from build123d import *

# Parameters (mm, degrees)
SKETCH1_W           = 65
SKETCH1_H           = 25
SKETCH1_R           = 4
BOSS_EXTRUDE1_DEPTH = 3
SKETCH2_W           = 36
SKETCH2_H           = 30
BOSS_EXTRUDE2_DEPTH = 25
CUT_EXTRUDE1_DEPTH  = 5
SKETCH4_R           = 5
CUT_EXTRUDE2_DEPTH  = 21
SKETCH6_R           = 1.2
SKETCH6_R_2         = 1.1
CUT_EXTRUDE4_DEPTH  = 26


with BuildPart() as part:
    # Sketch1 → Boss-Extrude1 (new body)
    with BuildSketch(Plane(origin=(0, 0, 0), x_dir=(1, 0, 0), z_dir=(0, 1, 0))):
        Rectangle(SKETCH1_W, SKETCH1_H)
        with Locations((-27.5, -7.5)):
            Circle(SKETCH1_R, mode=Mode.SUBTRACT)
        with Locations((27.119741523, 7.5)):
            Circle(SKETCH1_R, mode=Mode.SUBTRACT)
    extrude(amount=BOSS_EXTRUDE1_DEPTH)

    # Sketch2 → Boss-Extrude2 (add)
    with BuildSketch(Plane(origin=(0, 0, -12.5), x_dir=(-1, 0, 0), z_dir=(0, 0, -1))):
        with Locations((0, 18)):
            Rectangle(SKETCH2_W, SKETCH2_H)
    extrude(amount=-BOSS_EXTRUDE2_DEPTH)

    # Sketch3 → Cut-Extrude1 (cut)
    with BuildSketch(Plane(origin=(0, 0, -12.5), x_dir=(-1, 0, 0), z_dir=(0, 0, -1))):
        with BuildLine():
            Line((-15, 30), (15, 30))
            Line((15, 30), (15, 19.5))
            ThreePointArc((15, 19.5), (12.5, 17), (15, 14.5))
            Line((15, 14.5), (15, 4))
            Line((15, 4), (-15, 4))
            Line((-15, 4), (-15, 14.5))
            ThreePointArc((-15, 14.5), (-12.5, 17), (-15, 19.5))
            Line((-15, 19.5), (-15, 30))
        make_face()
    extrude(amount=-CUT_EXTRUDE1_DEPTH, mode=Mode.SUBTRACT)

    # Sketch4 → Cut-Extrude2 (cut, through all)
    with BuildSketch(Plane(origin=(0, 0, -7.5), x_dir=(-1, 0, 0), z_dir=(0, 0, -1))):
        with Locations((0, 17)):
            Circle(SKETCH4_R)
    extrude(amount=-CUT_EXTRUDE2_DEPTH, mode=Mode.SUBTRACT)

    # Sketch6 → Cut-Extrude4 (cut, through all)
    with BuildSketch(Plane(origin=(0, 0, -12.5), x_dir=(-1, 0, 0), z_dir=(0, 0, -1))):
        with Locations((-15, 17)):
            Circle(SKETCH6_R)
        with Locations((15, 17)):
            Circle(SKETCH6_R_2)
    extrude(amount=-CUT_EXTRUDE4_DEPTH, mode=Mode.SUBTRACT)


solid = part.part
Geometry check sheet. Reference: the model listing, model coordinates, mm. A direction names the side the tool comes from. Give positions to 0.01 mm unless a question says otherwise; leave off trailing zeros. Order: outer loops, then holes, each group sorted by start corner. A loop starts at its lowest first (then second) coordinate and runs counter-clockwise, first axis right, second up.
1) Cross-section at C-C (y = 17). Record the boundary of the cut face in (x, z), then the cut area to 3 significant figures.
Results are:
outline: (-18, -12.5) - (-16.1, -12.5) - (-16.1, 12.5) - (-18, 12.5) - close; (-13.9, -12.5) - (-12.5, -12.5) - (-12.5, -7.5) - (-5, -7.5) - (-5, 12.5) - (-13.9, 12.5) - close; (5, -7.5) - (12.5, -7.5) - (12.5, -12.5) - (13.8, -12.5) - (13.8, 12.5) - (5, 12.5) - close; (16.2, -12.5) - (18, -12.5) - (18, 12.5) - (16.2, 12.5) - close
area: 460 mm2
2) Cross-section at A-A (z = 7.5). Record the boundary of the cut face in (x, y), then the cut area to 3 significant figures.
Results are:
outline: (-32.5, 0) - (-31.5, 0) - (-31.5, 3) - (-32.5, 3) - close; (-23.5, 0) - (32.5, 0) - (32.5, 3) - (18, 3) - (18, 33) - (-18, 33) - (-18, 3) - (-23.5, 3) - close; hole circle Ø2.2 at (-15, 17); hole circle Ø10 at (0, 17); hole circle Ø2.4 at (15, 17)
area: 1,160 mm2
3) Cross-section at B-B (x = -27.5). Record the boundary of the cut face in (y, z), then the cut area to 3 significant figures.
Results are:
outline: (0, -12.5) - (3, -12.5) - (3, 3.5) - (0, 3.5) - close; (0, 11.5) - (3, 11.5) - (3, 12.5) - (0, 12.5) - close
area: 51.0 mm2
4) Cross-section at D-D (z = 2.5). Record the boundary of the cut face in (x, y).
Results are:
outline: (-32.5, 0) - (32.5, 0) - (32.5, 3) - (18, 3) - (18, 33) - (-18, 33) - (-18, 3) - (-32.5, 3) - close; hole circle Ø2.2 at (-15, 17); hole circle Ø10 at (0, 17); hole circle Ø2.4 at (15, 17)
5) Gauge pin test, flat ends, axial feed: pin 1 (5 mm diameter, centred on y = 22, z = 7.5, fed in from -X); pin 2 (1.8 mm diameter, centred on x = -15, y = 17, fed in from -Z); pin 3 (16 mm diameter, centred on x = 0, y = 17, fed in from -Z); pin 4 (7 mm diameter, centred on x = 23, z = -2.5, fed in from +Y). Record the tip position at first contact, or that the pin passes through.
Results are:
pin 1: stops at x = -18
pin 2: passes through
pin 3: stops at z = -7.5
pin 4: stops at y = 3
6) Tool access check on faces 4 (the flat face through (-18, 18, 0)), 5 (the flat face through (0, 33, 0)), 6 (the flat face through (0, 30, -10)), 7 (the flat face through (25, 3, 0)). Record the directions out of +Z, -Z, +X, -X, +Y, -Y that give a thin tool (end or side, any length) a straight path to the whole face; none if there is none.
Results are:
face 4: +Z, -Z, -X, +Y
face 5: +Z, -Z, +X, -X, +Y
face 6: -Z
face 7: +Z, -Z, +X, +Y
7) Material ranges on probe 1 along Y at (x, z) = (-15, 6.5); probe 2 along X at (y, z) = (0.6, -7.5); probe 3 along X at (y, z) = (1.55, 7.5), recorded low to high.
Results are:
probe 1: y = 0 to 15.9, 18.1 to 33
probe 2: x = -32.5 to 23.12, 31.12 to 32.5
probe 3: x = -32.5 to -31.5, -23.5 to 32.5
8) Draft check along Z on faces 1 (the cylindrical face through (1.08, 12.12, 2.36)), 2 (the cylindrical face through (-30.7, 1.5, 9.9)), 3 (the flat face through (0, 3, -12.5)). Enter one of: released by +Z, released by -Z, zero draft, split by the parting line, or undercut.
Results are:
face 1: zero draft
face 2: undercut
face 3: released by -Z
